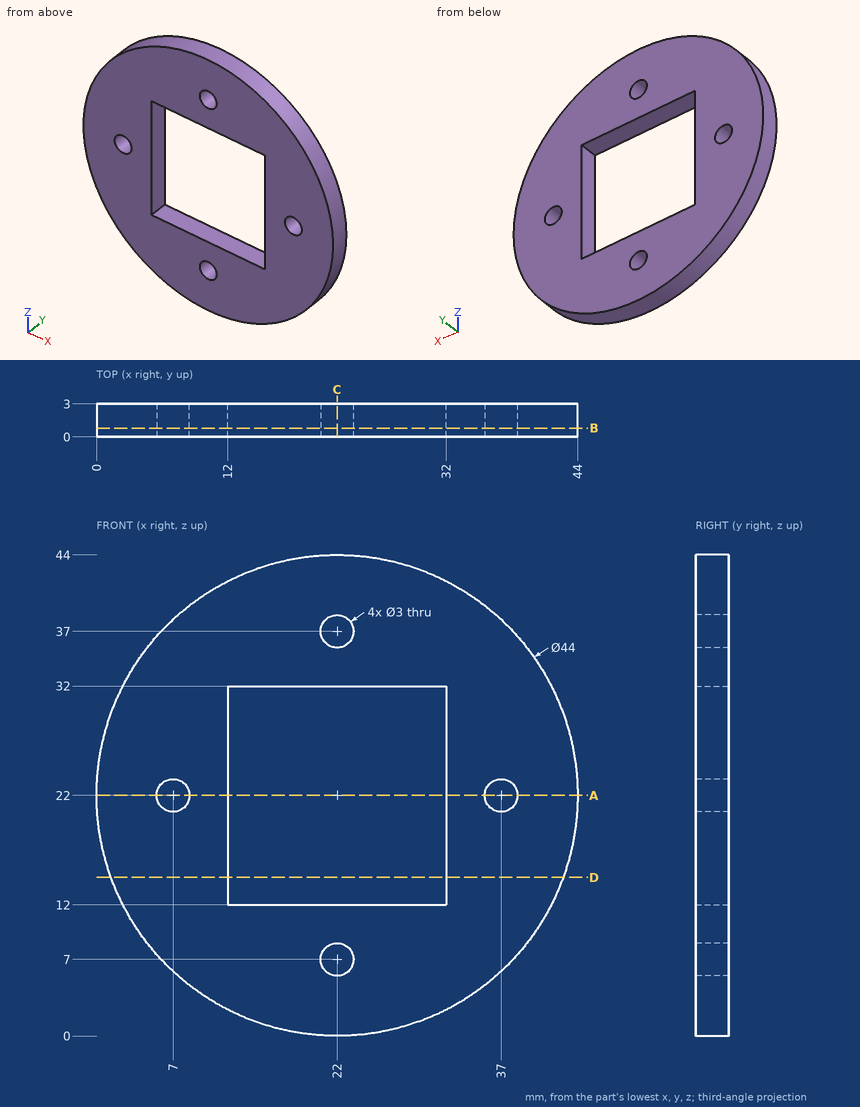
Verification items for this drawing (mm, ordinates from the low corner). Coordinates: 2 decimals unless noted, no trailing zeros. Order: outer loops, then holes, each group sorted by start corner. A loop starts at its lowest first (then second) coordinate and runs counter-clockwise, first axis right, second up. Notation, with made-up numbers: M 54,-9.5 L 95,-9.5 A23 ccw 95,18.5 Z; hole C -11.5,-30.75 d9. An arc over 180 degrees is marked long. Answer as a JSON object with one key per item and string values.
Q1. Cross-section at D-D on z = 14.5. Record the cut outline in (x, y), and give its area (3 significant figures).
Results are:
{"outline": "M 1.32,0 L 12,0 L 12,3 L 1.32,3 Z; M 32,0 L 42.68,0 L 42.68,3 L 32,3 Z", "area": "64.1 mm²"}
Q2. Cross-section at C-C on x = 22. Record the cut outline in (y, z).
Results are:
{"outline": "M 0,0 L 3,0 L 3,5.5 L 0,5.5 Z; M 0,8.5 L 3,8.5 L 3,12 L 0,12 Z; M 0,32 L 3,32 L 3,35.5 L 0,35.5 Z; M 0,38.5 L 3,38.5 L 3,44 L 0,44 Z"}
Q3. Cross-section at B-B on y = 0.8. Record the cut outline in (x, z).
Results are:
{"outline": "C 22,22 d44; hole C 7,22 d3; hole M 12,12 L 32,12 L 32,32 L 12,32 Z; hole C 22,7 d3; hole C 22,37 d3; hole C 37,22 d3"}
Q4. Depth check by flat-ended pin: pin 1 Ø4 at (x, z) = (7, 22) entering from -Y; pin 2 Ø0.9 at (x, y) = (22.5, 1.5) entering from +Z. Enter the tip coordinate at first touch or a pass-through.
Results are:
{"pin 1": "stops at y = 0", "pin 2": "stops at z = 44"}
Q5. Cross-section at A-A on z = 22. Record the cut outline in (x, y), and give its area (3 significant figures).
Results are:
{"outline": "M 0,0 L 5.5,0 L 5.5,3 L 0,3 Z; M 8.5,0 L 12,0 L 12,3 L 8.5,3 Z; M 32,0 L 35.5,0 L 35.5,3 L 32,3 Z; M 38.5,0 L 44,0 L 44,3 L 38.5,3 Z", "area": "54.0 mm²"}
Q6. Scan lines: line 1 (X direction, y = 2.1, z = 22); line 2 (X direction, y = 1.1, z = 31.5). Record each from-to range of solid material in increasing order.
Results are:
{"line 1": "x = 0 to 5.5, 8.5 to 12, 32 to 35.5, 38.5 to 44", "line 2": "x = 2.16 to 12, 32 to 41.84"}
